Part model, mm, in its own coordinate system. Face numbers are marked on the shaded views. A direction names the side the tool comes from. Round coordinates to 2 decimals unless told otherwise and drop trailing zeros. Write each loop counter-clockwise with the first axis right and the second up, starting at its lowest first coordinate (ties: lowest second). Pieces come first, ordered by that corner, then holes. Notation, with made-up numbers: (-11, -30) -> (39, -30) arc R13 cw to (39, -17) -> close; hole circle Ø2 at (-12.5, -32.75). An arc over 180 degrees is marked (long way). Return JSON: item names as keys, results as strings. Group by question number.
(1) Mould opens along Y. For the marked faces 3, 4, 5 and 6 say: +Y half, -Y half, draft (parallel to the pull), parting line (faces both ways), or undercut.
(2) Tool access for the marked faces 1 and 2: list every direction of +Z, -Z, +X, -X, +Y, -Y with a clear straight run to the whole face (end or side of a thin tool).
(3) Drop flat-ended pins along their axis: pin 1 Ø10 at (y, z) = (40.1, 10) entering from -X; pin 2 Ø12 at (x, y) = (68, 102.5) entering from +Z. Give the stop position or say it passes through.
(4) Saw through at C-C (z = 2). List the corners of the cut face in (x, y), plus the area to 3 significant figures.
(5) Drill centre lines: L1, parallel to Y at x = -62.5, z = 10; L2, parallel to Y at x = -54.25, z = 10; L3, parallel to Y at x = -56, z = 10. Where is each one in solid material? Low to high. Write a range as from..to.
(6) Saw through at D-D (y = 28). List the corners of the cut face in (x, z), plus the area to 3 significant figures.
(7) Saw through at A-A (x = 48). List the corners of the cut face in (y, z).
(8) Saw through at B-B (y = 93). List the corners of the cut face in (x, z).
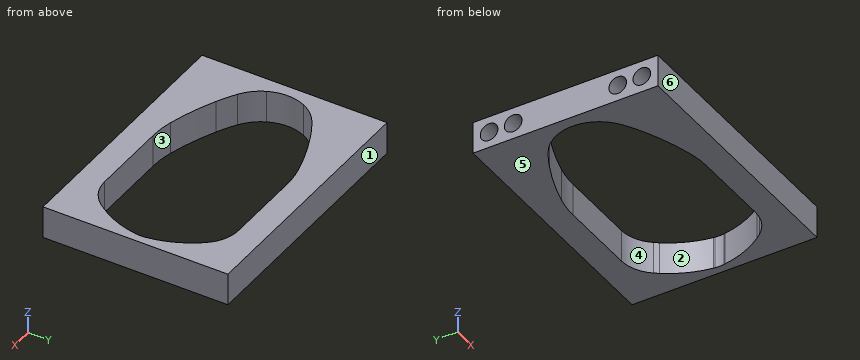
from build123d import *

# Parameters (mm, degrees)
SKETCH_4_W          = 160
SKETCH_4_H          = 115
EXTRUDE_1_DEPTH     = 20
CUT_EXTRUDE_1_DEPTH = 20
SKETCH_16_R         = 5.5
CUT_EXTRUDE_2_DEPTH = 15


with BuildPart() as part:
    # 草圖4 → 填料-伸長1 (new body)
    with BuildSketch(Plane.XY):
        with Locations((14.659712787, 72.59909222)):
            Rectangle(SKETCH_4_W, SKETCH_4_H)
    extrude(amount=EXTRUDE_1_DEPTH)

    # 草圖2 → 除料-伸長1 (cut)
    with BuildSketch(Plane.XY):
        with BuildLine():
            Line((9.582154386, 114.239387395), (32.639572719, 114.239387395))
            Line((32.639572719, 114.239387395), (35.911975242, 114.239387395))
            Line((35.911975242, 114.239387395), (58.302252446, 114.239387395))
            ThreePointArc((58.302252446, 114.239387395), (68.354977159, 111.933757574), (76.3981894, 105.477757274))
            ThreePointArc((76.3981894, 105.477757274), (77.386875553, 104.202213525), (78.350890948, 102.907923572))
            ThreePointArc((78.350890948, 102.907923572), (85.469179447, 90.183153699), (89.343429579, 76.126838912))
            Line((89.343429579, 76.126838912), (89.450916797, 75.407862922))
            ThreePointArc((89.450916797, 75.407862922), (89.659712787, 72.59909222), (89.450916797, 69.790321519))
            Line((89.450916797, 69.790321519), (89.343429579, 69.071345528))
            ThreePointArc((89.343429579, 69.071345528), (85.469179447, 55.015030741), (78.350890948, 42.290260868))
            ThreePointArc((78.350890948, 42.290260868), (77.386875553, 40.995970915), (76.3981894, 39.720427166))
            ThreePointArc((76.3981894, 39.720427166), (68.354977159, 33.264426866), (58.302252446, 30.958797045))
            Line((58.302252446, 30.958797045), (35.911975242, 30.958797045))
            Line((35.911975242, 30.958797045), (32.639572719, 30.958797045))
            Line((32.639572719, 30.958797045), (9.582154386, 30.958797045))
            ThreePointArc((9.582154386, 30.958797045), (2.328045496, 31.402381927), (-4.817967678, 32.726526576))
            ThreePointArc((-4.817967678, 32.726526576), (-19.619782039, 37.212171907), (-33.900352311, 43.151871824))
            ThreePointArc((-33.900352311, 43.151871824), (-39.787433986, 46.173940455), (-45.481740166, 49.545217155))
            ThreePointArc((-45.481740166, 49.545217155), (-51.391366265, 54.573313812), (-55.677619443, 61.041193705))
            ThreePointArc((-55.677619443, 61.041193705), (-58.292337425, 72.59909222), (-55.677619443, 84.156990735))
            ThreePointArc((-55.677619443, 84.156990735), (-51.391366265, 90.624870628), (-45.481740166, 95.652967285))
            ThreePointArc((-45.481740166, 95.652967285), (-39.787433986, 99.024243985), (-33.900352311, 102.046312617))
            ThreePointArc((-33.900352311, 102.046312617), (-19.619782039, 107.986012534), (-4.817967678, 112.471657865))
            ThreePointArc((-4.817967678, 112.471657865), (2.328045496, 113.795802514), (9.582154386, 114.239387395))
        make_face()
    extrude(amount=CUT_EXTRUDE_1_DEPTH, mode=Mode.SUBTRACT)

    # 草圖16 → 除料-伸長2 (cut)
    with BuildSketch(Plane(origin=(-66.2, 0, 0), x_dir=(0, 0, -1), z_dir=(1, 0, 0))):
        with Locations((-10, 120.09909222)):
            Circle(SKETCH_16_R)
        with Locations((-10, 105.09909222)):
            Circle(SKETCH_16_R)
        with Locations((-10, 40.09909222)):
            Circle(SKETCH_16_R)
        with Locations((-10, 25.09909222)):
            Circle(SKETCH_16_R)
    extrude(amount=CUT_EXTRUDE_2_DEPTH, mode=Mode.SUBTRACT)


solid = part.part
Computed values:
{
 "1": {"face 3": "undercut", "face 4": "undercut", "face 5": "draft", "face 6": "-Y half"},
 "2": {"face 1": "+Z, -Z, +X, -X, +Y", "face 2": "+Z, -Z"},
 "3": {"pin 1": "x = -51.2", "pin 2": "through"},
 "4": {"outline": "(-65.34, 15.1) -> (94.66, 15.1) -> (94.66, 130.1) -> (-65.34, 130.1) -> close; hole (-55.68, 61.04) arc R27.75 ccw to (-45.48, 49.55) arc R109.78 ccw to (-33.9, 43.15) arc R154.87 ccw to (-4.82, 32.73) arc R59.54 ccw to (9.58, 30.96) -> (58.3, 30.96) arc R23.07 ccw to (76.4, 39.72) arc R84.06 ccw to (78.35, 42.29) arc R60.62 ccw to (89.34, 69.07) -> (89.45, 69.79) arc R19 ccw to (89.45, 75.41) -> (89.34, 76.13) arc R60.62 ccw to (78.35, 102.91) arc R84.06 ccw to (76.4, 105.48) arc R23.07 ccw to (58.3, 114.24) -> (9.58, 114.24) arc R59.54 ccw to (-4.82, 112.47) arc R154.87 ccw to (-33.9, 102.05) arc R109.78 ccw to (-45.48, 95.65) arc R27.75 ccw to (-55.68, 84.16) arc R26.85 ccw to start", "area": "8,110 mm2"},
 "5": {"L1": "15.1..19.6, 30.6..34.6, 45.6..99.6, 110.6..114.6, 125.6..130.1", "L2": "15.1..19.6, 30.6..34.6, 45.6..58.42, 86.78..99.6, 110.6..114.6, 125.6..130.1", "L3": "15.1..19.6, 30.6..34.6, 45.6..61.74, 83.46..99.6, 110.6..114.6, 125.6..130.1"},
 "6": {"outline": "(-65.34, 0) -> (94.66, 0) -> (94.66, 20) -> (-65.34, 20) -> (-65.34, 14.67) -> (-51.2, 14.67) -> (-51.2, 5.33) -> (-65.34, 5.33) -> close", "area": "3,070 mm2"},
 "7": {"outline": "(15.1, 0) -> (30.96, 0) -> (30.96, 20) -> (15.1, 20) -> close; (114.24, 0) -> (130.1, 0) -> (130.1, 20) -> (114.24, 20) -> close"},
 "8": {"outline": "(-65.34, 0) -> (-49.01, 0) -> (-49.01, 20) -> (-65.34, 20) -> close; (84.23, 0) -> (94.66, 0) -> (94.66, 20) -> (84.23, 20) -> close"}
}
